```python
from build123d import *

# Parameters (mm, degrees)
F0_R     = 40
F0_R_2   = 34
F0_R_3   = 32.5
F1_DEPTH = 3
F2_R     = 34
F2_R_2   = 32.5
F3_DEPTH = 27
F4_W     = 1
F4_H     = 46
F5_DEPTH = 56.9


with BuildPart() as f1:
    # F0 (on Front) → F1 (new body)
    with BuildSketch(Plane.XZ):
        with Locations((-117.890202, 35.398554)):
            Circle(F0_R)
        with Locations((-117.890202, 35.398554)):
            Circle(F0_R_2, mode=Mode.SUBTRACT)
        with Locations((-117.890202, 35.398554)):
            Circle(F0_R_2)
        with Locations((-117.890202, 35.398554)):
            Circle(F0_R_3, mode=Mode.SUBTRACT)
    extrude(amount=F1_DEPTH)

    # F2 (on face) → F3 (join)
    with BuildSketch(Plane.XZ.offset(3)):
        with Locations((-117.890202, 35.398554)):
            Circle(F2_R)
        with Locations((-117.890202, 35.398554)):
            Circle(F2_R_2, mode=Mode.SUBTRACT)
    extrude(amount=F3_DEPTH)

    # F4 (on face) → F5 (cut)
    with BuildSketch(Plane.XZ.offset(30)):
        with Locations((-117.390202, 12.398554)):
            Rectangle(F4_W, F4_H)
    extrude(amount=-F5_DEPTH, mode=Mode.SUBTRACT)


solid = f1.part
```
Can you work these out from the model? Positions are in its coordinate system, mm. A direction names the side the tool comes from. Coordinates: 2 decimals unless noted, no trailing zeros. Write each loop counter-clockwise with the first axis right and the second up, starting at its lowest first coordinate (ties: lowest second). Pieces come first, ordered by that corner, then holes. Notation, with made-up numbers: M 10,15 L 43,15 A21 ccw 43,50 Z; hole C 67,-15 d8. An arc over 180 degrees is marked long. Write item = value, one per line. Start each with the question number.
Q1. On a 3-axis mill with a long thin cutter (end or side, diameter ignored), from which of +Z, -Z, +X, -X, +Y, -Y can I reach the whole of each face in a straight line? I mean faces 1 (the face through (-117.89, -12, 2)), 2 (the face through (-118.1, 0, 68.2)), 3 (the face through (-136, -3, 6)). Say none if no direction works.
Q2. If I drill on L1, parallel to Z at x = -118, y = -24.25; L2, parallel to Z at x = -98.5, y = -10; L3, parallel to X at y = -20.75, z = 25, over which ranges is the centre line in solid material (lowest first)? Write a range as [from, to].
Q3. If we section it at A-A, the plane x = -141.5: Write out the boundary of the cut face in (y, z).
Q4. I'm going to push flat-ended pins straight in: pin 1 (6 mm diameter, centred on x = -143.5, y = -14.5, fed in from +Z); pin 2 (12 mm diameter, centred on y = -11, z = 47.5, fed in from -X); pin 3 (1 mm diameter, centred on y = -19.5, z = 29.5, fed in from -X); pin 4 (8 mm diameter, centred on x = -146.5, z = 32.5, fed in from +Y). Where does each tip first touch, or does it pass through?
Q5. If we section it at B-B, the plane z = 26: Write out the boundary of the cut face in (x, y).
Q6. If we section it at C-C, the plane y = -9.25: Write out the boundary of the cut face in (x, z), then the cut area to 3 significant figures.
Check sheet entries:
q1.face_1 = -Z, +Y, -Y
q1.face_2 = +Z, -Z, +X, -X, +Y
q1.face_3 = -Y
q2.L1 = [1.4, 2.9], [67.9, 69.4]
q2.L2 = [7.47, 9.32], [61.48, 63.33]
q2.L3 = [-150.26, -148.68], [-87.1, -85.52]
q3.outline = M -30,10.93 L -3,10.93 L -3,3.11 L 0,3.11 L 0,13.06 L -30,13.06 Z; M -30,57.73 L 0,57.73 L 0,67.69 L -3,67.69 L -3,59.86 L -30,59.86 Z
q4.pin_1 = 60.79
q4.pin_2 = -151.34
q4.pin_3 = -151.46
q4.pin_4 = 0
q5.outline = M -156.77,-3 L -150.57,-3 L -150.57,-30 L -149,-30 L -149,0 L -156.77,0 Z; M -86.78,-30 L -85.22,-30 L -85.22,-3 L -79.01,-3 L -79.01,0 L -86.78,0 Z
q6.outline = M -117.89,1.4 L -117.89,2.9 A32.5 cw long -116.89,2.91 L -116.89,1.41 A34 ccw long Z
q6.area = 312 mm²
